CAD build for the part. Positions are in the model's coordinates, mm. A direction names the side the tool comes from. Round coordinates to 2 decimals unless told otherwise and drop trailing zeros. Order: outer loops, then holes, each group sorted by start corner. A loop starts at its lowest first (then second) coordinate and runs counter-clockwise, first axis right, second up. Notation, with made-up numbers: M -22,14.5 L 37,14.5 A26 ccw 37,40.5 Z; hole C -15.75,77.5 d11. An arc over 180 degrees is marked long. Answer as a JSON object with one key per item and string values.
```python
from build123d import *

# Parameters (mm, degrees)
F0_W     = 2
F0_H     = 2
F1_DEPTH = 5


with BuildPart() as f1:
    # F0 (on Front) → F1 (new body)
    with BuildSketch(Plane.XZ):
        Rectangle(F0_W, F0_H)
        with Locations((2, 0)):
            Rectangle(F0_W, F0_H)
        with Locations((-2, 0)):
            Rectangle(F0_W, F0_H)
        with Locations((4, 0)):
            Rectangle(F0_W, F0_H)
        Polygon((3, 3), (3, 1), (5, 1), (5, 2.5), (5, 3), (4.5, 3), align=None)
        Polygon((-5, 1), (-3, 1), (-3, 3), (-4, 3), (-4.5, 3), (-5, 3), (-5, 2.5), (-5, 2), align=None)
        with Locations((-4, 0)):
            Rectangle(F0_W, F0_H)
        with Locations((6, 0)):
            Rectangle(F0_W, F0_H)
        with Locations((-6, 0)):
            Rectangle(F0_W, F0_H)
        with Locations((6, -2)):
            Rectangle(F0_W, F0_H)
        with Locations((2, -6)):
            Rectangle(F0_W, F0_H)
        with Locations((0, -6)):
            Rectangle(F0_W, F0_H)
        Polygon((5, 3), (5, 2.5), (5.5, 3), align=None)
        Polygon((5, 3.5), (4.5, 3), (5, 3), align=None)
        with Locations((-2, -6)):
            Rectangle(F0_W, F0_H)
        with Locations((-6, -2)):
            Rectangle(F0_W, F0_H)
        with Locations((6, -4)):
            Rectangle(F0_W, F0_H)
        with Locations((4, -6)):
            Rectangle(F0_W, F0_H)
        with Locations((8, -2)):
            Rectangle(F0_W, F0_H)
        Polygon((5, 3.5), (5, 3), (5.5, 3), (7, 3), (7, 5), (5, 5), align=None)
        with Locations((-4, -6)):
            Rectangle(F0_W, F0_H)
        with Locations((-6, -4)):
            Rectangle(F0_W, F0_H)
        with Locations((-8, -2)):
            Rectangle(F0_W, F0_H)
        Polygon((-5, 3), (-4.5, 3), (-5, 3.5), align=None)
        Polygon((-5.5, 3), (-5, 2.5), (-5, 3), align=None)
        with Locations((8, -4)):
            Rectangle(F0_W, F0_H)
        with Locations((6, -6)):
            Rectangle(F0_W, F0_H)
        with Locations((-6, -6)):
            Rectangle(F0_W, F0_H)
        with Locations((-8, -4)):
            Rectangle(F0_W, F0_H)
        Polygon((-5.5, 3), (-5, 3), (-5, 3.5), (-5, 4), (-5, 5), (-7, 5), (-7, 3), (-6, 3), align=None)
        with Locations((10, -4)):
            Rectangle(F0_W, F0_H)
        Polygon((7, -7), (5, -7), (5, -8.5), (5, -9), (5.5, -9), (7, -9), align=None)
        Polygon((-5, -8), (-5, -7), (-7, -7), (-7, -9), (-6, -9), (-5.5, -9), (-5, -9), (-5, -8.5), align=None)
        with Locations((-10, -4)):
            Rectangle(F0_W, F0_H)
        with Locations((10, -6)):
            Rectangle(F0_W, F0_H)
        Polygon((5, -9), (5, -8.5), (4.5, -9), align=None)
        with Locations((-10, -6)):
            Rectangle(F0_W, F0_H)
        with Locations((10, -8)):
            Rectangle(F0_W, F0_H)
        Polygon((5, -9.5), (5, -9), (4.5, -9), (3, -9), (3, -11), (5, -11), align=None)
        Polygon((5.5, -9), (5, -9), (5, -9.5), align=None)
        Polygon((-4.5, -9), (-5, -8.5), (-5, -9), align=None)
        with Locations((-10, -8)):
            Rectangle(F0_W, F0_H)
        with Locations((2, -10)):
            Rectangle(F0_W, F0_H)
        Polygon((-4.5, -9), (-5, -9), (-5, -9.5), (-5, -10), (-5, -11), (-3, -11), (-3, -9), (-4, -9), align=None)
        Polygon((-5, -9.5), (-5, -9), (-5.5, -9), align=None)
        with Locations((-2, -10)):
            Rectangle(F0_W, F0_H)
        with Locations((-2, -2)):
            Rectangle(F0_W, F0_H)
        with Locations((-4, -4)):
            Rectangle(F0_W, F0_H)
        with Locations((-2, -4)):
            Rectangle(F0_W, F0_H)
        with Locations((0, -4)):
            Rectangle(F0_W, F0_H)
        with Locations((0, -2)):
            Rectangle(F0_W, F0_H)
        with Locations((4, -4)):
            Rectangle(F0_W, F0_H)
        with Locations((2, -4)):
            Rectangle(F0_W, F0_H)
        with Locations((2, -2)):
            Rectangle(F0_W, F0_H)
    extrude(amount=F1_DEPTH)


solid = f1.part
```
Item 1: Saw through at C-C on z = -2.75. List the corners of the cut face in (x, y), and give its area (3 significant figures).
Worked answers:
{"outline": "M -9,-5 L -5,-5 L -5,0 L -9,0 Z; M -3,-5 L 3,-5 L 3,0 L -3,0 Z; M 5,-5 L 9,-5 L 9,0 L 5,0 Z", "area": "70.0 mm2"}
Item 2: Wall check: line 1 along X through (y, z) = (-0.5, -8); line 2 along Z through (x, y) = (-3.25, -1.35); line 3 along X through (y, z) = (-2.15, -5.5). Give the ranges that are in metal, low to high. Write a range as [from, to].
Worked answers:
{"line 1": "x = [-11, -9], [-7, -5], [5, 7], [9, 11]", "line 2": "z = [-11, -9], [-7, -3], [-1, 3]", "line 3": "x = [-11, -9], [-7, 7], [9, 11]"}
Item 3: Two-plate mould, pull along X, no slides. Class faces 5 (the flat face through (0, 0, -5)), 6 (the flat face through (3, -2, -2)), 7 (the flat face through (-11, -2, -6)): released by +X, released by -X, zero draft, split by the parting line, or undercut.
Worked answers:
{"face 5": "zero draft", "face 6": "undercut", "face 7": "released by -X"}
Item 4: Saw through at A-A on z = -6. List the corners of the cut face in (x, y), and give its area (3 significant figures).
Worked answers:
{"outline": "M -11,-5 L -9,-5 L -9,0 L -11,0 Z; M -7,-5 L 7,-5 L 7,0 L -7,0 Z; M 9,-5 L 11,-5 L 11,0 L 9,0 Z", "area": "90.0 mm2"}
Item 5: Drop flat-ended pins along their axis: pin 1 Ø2 at (x, z) = (-1.5, 0) entering from +Y; pin 2 Ø1.6 at (y, z) = (-2, -0.5) entering from +X; pin 3 Ø1.6 at (y, z) = (-3, -10.5) entering from -X; pin 4 Ø0.6 at (y, z) = (-3.5, 0) entering from -X. Give the stop position or say it passes through.
Worked answers:
{"pin 1": "stops at y = 0", "pin 2": "stops at x = 9", "pin 3": "stops at x = -5", "pin 4": "stops at x = -7"}
Item 6: 3-axis set-ups, long thin cutter, end or side, ignore diameter. For faces 1 (the flat face through (5, -2, 4)), 2 (the flat face through (9, -2, -7)), 3 (the flat face through (4, -2, -1)), 4 (the flat face through (-7, -2, 0)): which of +Z, -Z, +X, -X, +Y, -Y reach the whole face in a straight line?
Worked answers:
{"face 1": "+Z, +Y, -Y", "face 2": "-Z, +Y, -Y", "face 3": "+Y, -Y", "face 4": "+Z, -X, +Y, -Y"}
Item 7: Saw through at D-D on x = 2.5. List the corners of the cut face in (y, z), and give its area (3 significant figures).
Worked answers:
{"outline": "M -5,-11 L 0,-11 L 0,-9 L -5,-9 Z; M -5,-7 L 0,-7 L 0,1 L -5,1 Z", "area": "50.0 mm2"}
Item 8: Saw through at B-B on x = 6.5. List the corners of the cut face in (y, z).
Worked answers:
{"outline": "M -5,-9 L 0,-9 L 0,1 L -5,1 Z; M -5,3 L 0,3 L 0,5 L -5,5 Z"}
